```python
from build123d import *

# Parameters (mm, degrees)
F3_DEPTH = 2


with BuildPart() as f1:
    # F0 (on Front) → F1 (revolve)
    with BuildSketch(Plane.XZ):
        with BuildLine():
            Line((-10.2, 0), (0, 0))
            Line((0, 0), (0, 2))
            Line((0, 2), (-8, 2))
            Line((-8, 2), (-8, 3.8))
            Line((-8, 3.8), (-8.677624, 3.8))
            ThreePointArc((-8.677624, 3.8), (-9.72023, 2.954011), (-10.2, 1.7))
            Line((-10.2, 1.7), (-10.2, 0))
        make_face()
    revolve(axis=Axis((-5.1, 0, 0), (1, 0, 0)))

    # F2 (on face) → F3 (cut)
    with BuildSketch(Plane(origin=(-10.2, 0, 0), x_dir=(0, -1, 0), z_dir=(-1, 0, 0))):
        Polygon((0.721688, 1.25), (-0.721688, 1.25), (-1.443376, 0), (-0.721688, -1.25), (0.721688, -1.25), (1.443376, 0), align=None)
    extrude(amount=-F3_DEPTH, mode=Mode.SUBTRACT)


solid = f1.part
```
Build history of the part. All positions in model axes, mm. A direction names the side the tool comes from. Round coordinates to 2 decimals unless told otherwise and drop trailing zeros. Write each loop counter-clockwise with the first axis right and the second up, starting at its lowest first coordinate (ties: lowest second). Pieces come first, ordered by that corner, then holes.
1) Drill centre lines: probe 1 along X at (y, z) = (-0.25, -0.5); probe 2 along Z at (x, y) = (-9.5, 2.75); probe 3 along X at (y, z) = (2.5, 1.75). Where is each one in solid material? Low to high.
2) Band-saw the part on A-A, the plane x = -6. List the corners of the cut face in (y, z), and give its area (3 significant figures).
3) Pin check, flat tips, straight feed: pin 1 (2 mm diameter, centred on x = -7.5, z = 1.5, fed in from +Y); pin 2 (2.5 mm diameter, centred on y = 0.5, z = 0, fed in from +X); pin 3 (1.2 mm diameter, centred on y = 0.5, z = 0, fed in from -X); pin 4 (1.6 mm diameter, centred on x = -9.5, y = -0.5, fed in from +Z). Stop position of each tip, or through.
4) Mould opens along Z. For faces 1 (the flat face through (-8.2, 0, 0)), 2 (the flat face through (-8, 2, -2)), 3 (the cylindrical face through (-8.344, -0.167, -3.796)) say: +Z half, -Z half, draft (parallel to the pull), parting line (faces both ways), or undercut.
5) 3-axis set-ups, long thin cutter, end or side, ignore diameter. For faces 4 (the cylindrical face through (-4, 2, 0)), 5 (the flat face through (0, 0, 0)), 6 (the flat face through (-9, 0, 1.25)): which of +Z, -Z, +X, -X, +Y, -Y reach the whole face in a straight line?
Ans:
1. probe 1: x = -8.2 to 0
1. probe 2: z = -1.67 to 1.67
1. probe 3: x = -9.65 to -8
2. outline: circle Ø4 at (0, 0)
2. area: 12.6 mm2
3. pin 1: stops at y = 3.75
3. pin 2: stops at x = 0
3. pin 3: stops at x = -8.2
3. pin 4: stops at z = 3.77
4. face 1: undercut
4. face 2: draft
4. face 3: parting line
5. face 4: +X
5. face 5: +Z, -Z, +X, +Y, -Y
5. face 6: -X
